Source: three-view drawing plus pictorial views. Frame: mm from the lowest corner of the part. Round coordinates to 2 decimals unless told otherwise and drop trailing zeros. Loops run counter-clockwise (first coordinate to the right, second up) from the corner with the lowest first, then second, coordinate; pieces in that order, holes last. Notation, with made-up numbers: M 22,72 L 28,72 A14 ccw 28,99 Z; hole C 75.25,30 d2. An arc over 180 degrees is marked long. Answer as a JSON object with one key per item and string values.
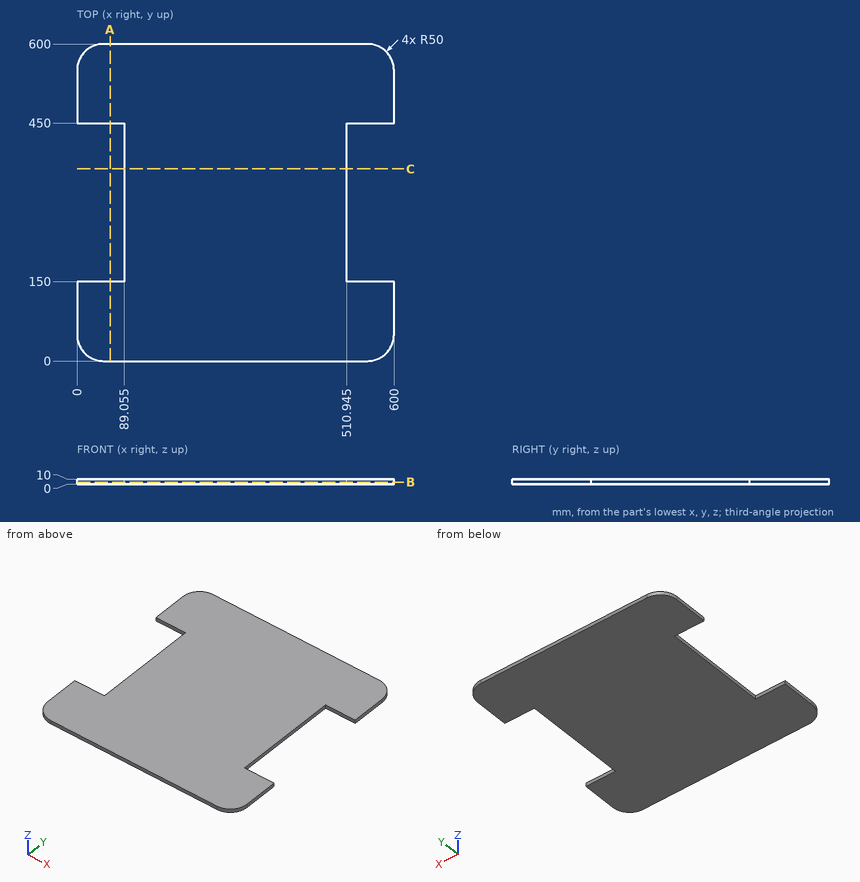
1) Cut plane C-C on y = 363.5. Return the cut outline in (x, z) (1 decimal), and give its area (3 significant figures).
Geometry results:
{"outline": "M 89.1,0 L 510.9,0 L 510.9,10 L 89.1,10 Z", "area": "4,220 mm2"}
2) Cut plane A-A on x = 62.5. Return the cut outline in (y, z), and give its area (3 significant figures).
Geometry results:
{"outline": "M 0,0 L 150,0 L 150,10 L 0,10 Z; M 450,0 L 600,0 L 600,10 L 450,10 Z", "area": "3,000 mm2"}
3) Cut plane B-B on z = 4. Return the cut outline in (x, y) (1 decimal).
Geometry results:
{"outline": "M 0,50 A50 ccw 50,0 L 550,0 A50 ccw 600,50 L 600,150 L 510.9,150 L 510.9,450 L 600,450 L 600,550 A50 ccw 550,600 L 50,600 A50 ccw 0,550 L 0,450 L 89.1,450 L 89.1,150 L 0,150 Z"}
4) Line query: probe 1 along Y at (x, z) = (62, 7.5); probe 2 along Y at (x, z) = (552.5, 8); probe 3 along X at (y, z) = (269.5, 7.5) (1 decimal). Output: solid intervals per line, ascending.
Geometry results:
{"probe 1": "0 to 150, 450 to 600", "probe 2": "0.06 to 150, 450 to 599.94", "probe 3": "89.1 to 510.9"}
5) First-contact query: pin 1 (5 mm diameter, centred on y = 196.5, z = 8, fed in from +X) (3 decimals); pin 2 (6 mm diameter, centred on x = 172.5, z = 5.5, fed in from -Y); pin 3 (2 mm diameter, centred on y = 176, z = 5.5, fed in from -X) (3 decimals). Flat tips, straight axial feed; report the tip coordinate or a pass-through.
Geometry results:
{"pin 1": "x = 510.945", "pin 2": "y = 0", "pin 3": "x = 89.055"}
